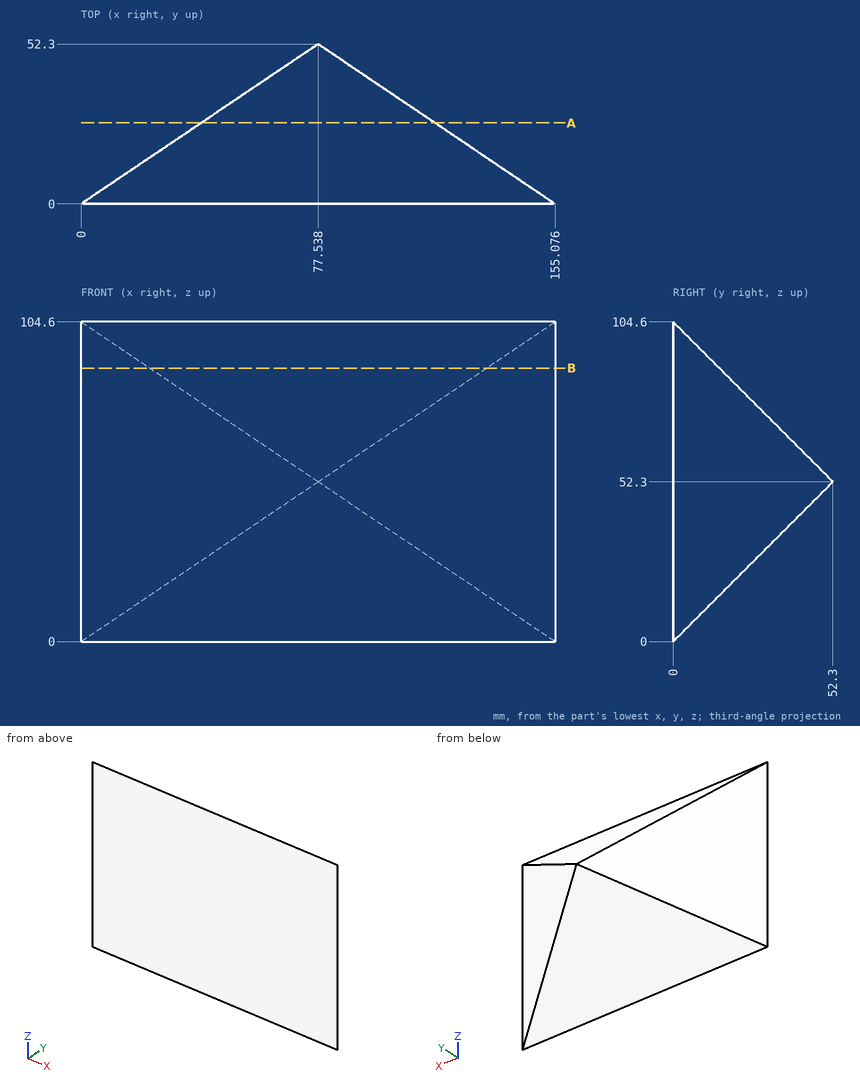
The figure shows three views and two pictorial views of one solid part (mm, origin at its lowest corner). Answer the questions. Coordinates: 2 decimals unless noted, no trailing zeros. Loops run counter-clockwise (first coordinate to the right, second up) from the corner with the lowest first, then second, coordinate; pieces in that order, holes last.
1) Find section A-A on y = 26.5. Write down the section's boundary in (x, z).
2) Flat-ended cylindrical pins translate along their axes: pin 1 Ø12 at (y, z) = (29, 70) entering from -X; pin 2 Ø8 at (y, z) = (13.5, 25.5) entering from +X; pin 3 Ø4 at (x, y) = (35.5, 17.5) entering from -Z. Find the tip coordinate at first contact, or state that the pin passes through.
3) Find section B-B on z = 89.5. Write down the section's boundary in (x, y), then the cut area to 3 significant figures.
4) Find the intervals of material crossed by L1, parallel to Y at x = 142, z = 29.5; L2, parallel to Z at x = 51, y = 28; L3, parallel to Y at x = 17, z = 56.5, in increasing order.
Values:
1. outline: (39.29, 26.5) - (115.79, 26.5) - (115.79, 78.1) - (39.29, 78.1) - close
2. pin 1: stops at x = 34.1
2. pin 2: stops at x = 140.99
2. pin 3: stops at z = 15.5
3. outline: (0, 0) - (155.08, 0) - (132.69, 15.1) - (22.39, 15.1) - close
3. area: 2,000 mm2
4. L1: y = 0 to 8.82
4. L2: z = 28 to 76.6
4. L3: y = 0 to 11.47
